Part model, mm, in its own coordinate system. A direction names the side the tool comes from. Round coordinates to 2 decimals unless told otherwise and drop trailing zeros. Loops run counter-clockwise (first coordinate to the right, second up) from the corner with the lowest first, then second, coordinate; pieces in that order, holes last. Notation, with made-up numbers: (57.25, 16.25) - (94.25, 16.25) arc R22 cw to (94.25, 50.25) - close; hole circle Ø1 at (60.5, 86.5). An arc over 180 degrees is marked (long way). Put each result on its own line as item: value.
from build123d import *

# Parameters (mm, degrees)
F1_DEPTH = 6.35


with BuildPart() as f1:
    # F0 (on Top) → F1 (new body)
    with BuildSketch(Plane.XY):
        with BuildLine():
            ThreePointArc((0, 11.049), (7.8128228253, 7.8128228253), (11.049, 0))
            ThreePointArc((11.049, 0), (7.8128228253, -7.8128228253), (0, -11.049))
            Line((0, -11.049), (0, -13.97))
            ThreePointArc((0, -13.97), (9.8782817332, -9.8782817332), (13.97, 0))
            ThreePointArc((13.97, 0), (9.8782817332, 9.8782817332), (0, 13.97))
            Line((0, 13.97), (0, 11.049))
        make_face()
        with BuildLine():
            ThreePointArc((0, -11.049), (-11.049, 0), (0, 11.049))
            Line((0, 11.049), (0, 13.97))
            ThreePointArc((0, 13.97), (-9.8782817332, 9.8782817332), (-13.97, 0))
            ThreePointArc((-13.97, 0), (-9.8782817332, -9.8782817332), (0, -13.97))
            Line((0, -13.97), (0, -11.049))
        make_face()
        with BuildLine():
            Line((0, 16.51), (0, 13.97))
            ThreePointArc((0, 13.97), (9.8782817332, 9.8782817332), (13.97, 0))
            Line((13.97, 0), (13.97, 30.48))
            ThreePointArc((13.97, 30.48), (9.8782817332, 20.6017182668), (0, 16.51))
        make_face()
        with BuildLine():
            ThreePointArc((-13.97, 0), (-9.8782817332, 9.8782817332), (0, 13.97))
            Line((0, 13.97), (0, 16.51))
            ThreePointArc((0, 16.51), (-9.8782817332, 20.6017182668), (-13.97, 30.48))
            Line((-13.97, 30.48), (-13.97, 0))
        make_face()
        with BuildLine():
            Line((0, -16.51), (0, -13.97))
            ThreePointArc((0, -13.97), (-9.8782817332, -9.8782817332), (-13.97, 0))
            Line((-13.97, 0), (-13.97, -30.48))
            ThreePointArc((-13.97, -30.48), (-9.8782817332, -20.6017182668), (0, -16.51))
        make_face()
        with BuildLine():
            ThreePointArc((13.97, 0), (9.8782817332, -9.8782817332), (0, -13.97))
            Line((0, -13.97), (0, -16.51))
            ThreePointArc((0, -16.51), (9.8782817332, -20.6017182668), (13.97, -30.48))
            Line((13.97, -30.48), (13.97, 0))
        make_face()
        with BuildLine():
            ThreePointArc((-13.97, 30.48), (-9.8782817332, 20.6017182668), (0, 16.51))
            ThreePointArc((0, 16.51), (9.8782817332, 20.6017182668), (13.97, 30.48))
            ThreePointArc((13.97, 30.48), (9.8782817459, 40.3582817204), (3.6e-08, 44.45))
            ThreePointArc((3.6e-08, 44.45), (-9.8782817204, 40.3582817459), (-13.97, 30.48))
        make_face()
        with BuildLine():
            ThreePointArc((11.049, 30.48), (7.8128228253, 22.6671771747), (0, 19.431))
            ThreePointArc((0, 19.431), (-7.8128228253, 38.2928228253), (11.049, 30.48))
        make_face(mode=Mode.SUBTRACT)
        with BuildLine():
            ThreePointArc((13.97, -30.48), (9.8782817332, -20.6017182668), (0, -16.51))
            ThreePointArc((0, -16.51), (-9.8782817332, -20.6017182668), (-13.97, -30.48))
            ThreePointArc((-13.97, -30.48), (-9.8782817062, -40.3582817602), (7.63e-08, -44.45))
            ThreePointArc((7.63e-08, -44.45), (9.8782817602, -40.3582817062), (13.97, -30.48))
        make_face()
        with BuildLine():
            ThreePointArc((11.049, -30.48), (-7.8128228253, -38.2928228253), (0, -19.431))
            ThreePointArc((0, -19.431), (7.8128228253, -22.6671771747), (11.049, -30.48))
        make_face(mode=Mode.SUBTRACT)
        with BuildLine():
            ThreePointArc((3.6e-08, 44.45), (9.8782817459, 40.3582817204), (13.97, 30.48))
            ThreePointArc((13.97, 30.48), (23.1619287876, 34.4165277907), (32.3538575753, 30.48))
            ThreePointArc((32.3538575753, 30.48), (17.6205349119, 40.808323286), (3.6e-08, 44.45))
        make_face()
        with BuildLine():
            ThreePointArc((32.3538575753, -30.48), (23.1619287876, -34.4165277907), (13.97, -30.48))
            ThreePointArc((13.97, -30.48), (9.8782817602, -40.3582817062), (7.63e-08, -44.45))
            ThreePointArc((7.63e-08, -44.45), (17.6205349304, -40.808323278), (32.3538575753, -30.48))
        make_face()
        with BuildLine():
            ThreePointArc((7.63e-08, -44.45), (-9.8782817062, -40.3582817602), (-13.97, -30.48))
            ThreePointArc((-13.97, -30.48), (-23.1619287876, -34.4165277907), (-32.3538575753, -30.48))
            ThreePointArc((-32.3538575753, -30.48), (-17.6205348604, -40.8083233083), (7.63e-08, -44.45))
        make_face()
        with BuildLine():
            ThreePointArc((-32.3538575753, 30.48), (-23.1619287876, 34.4165277907), (-13.97, 30.48))
            ThreePointArc((-13.97, 30.48), (-9.8782817204, 40.3582817459), (3.6e-08, 44.45))
            ThreePointArc((3.6e-08, 44.45), (-17.6205348789, 40.8083233003), (-32.3538575753, 30.48))
        make_face()
    extrude(amount=F1_DEPTH)


solid = f1.part
1. Pin check, flat tips, straight feed: P1, Ø2, axis at y = -14.5, z = 3, coming from the +X side; P2, Ø1.5, axis at x = 11.5, z = 4, coming from the +Y side; P3, Ø5, axis at x = 7.5, y = 34, coming from the +Z side; P4, Ø1, axis at x = 18, z = 5.5, coming from the -Y side. Stop position of each tip, or through.
A:
P1: stops at x = 13.97
P2: stops at y = 43.13
P3: passes through
P4: stops at y = -40.86
2. Probe line 1 along Y through (x, z) = (-2.5, 1); line 2 along X through (y, z) = (-32.5, 3); line 3 along Y through (x, z) = (-9.5, 4). List the from-to ranges inside material, lowest first. Write a range as [from, to].
A:
line 1: y = [-44.38, -41.24], [-19.72, -10.76], [10.76, 19.72], [41.24, 44.38]
line 2: x = [-30.32, -29.87], [-16.45, -10.86], [10.86, 16.45], [29.87, 30.32]
line 3: y = [-43.42, -36.12], [-24.84, -5.64], [5.64, 24.84], [36.12, 43.42]
3. Band-saw the part on A-A (y = 5). List the corners of the cut face in (x, z), plus the area to 3 significant figures.
A:
outline: (-13.97, 0) - (-9.85, 0) - (-9.85, 6.35) - (-13.97, 6.35) - close; (9.85, 0) - (13.97, 0) - (13.97, 6.35) - (9.85, 6.35) - close
area: 52.3 mm²
4. Two-plate mould, pull along Y, no slides. Class faces 1 (the flat face through (13.97, 0, 3)), 2 (the cylindrical face through (23.018, 34.416, 3.131)), 3 (the flat face through (-10, -6, 0)): pulls with the +Y half, pulls with the -Y half, needs draft (parallel to the pull), parting line crosses it, or undercut.
A:
face 1: undercut
face 2: undercut
face 3: needs draft
5. Tool access for faces 4 (the flat face through (-13.97, 0, 3)), 5 (the flat face through (-10, -6, 6.35)), 6 (the cylindrical face through (23.306, -34.416, 3.131)): list every direction of +Z, -Z, +X, -X, +Y, -Y with a clear straight run to the whole face (end or side of a thin tool).
A:
face 4: +Z, -Z, -X
face 5: +Z, +X, -X, +Y, -Y
face 6: +Z, -Z
6. Band-saw the part on C-C (y = -32). List the corners of the cut face in (x, z), plus the area to 3 significant figures.
A:
outline: (-30.85, 0) - (-30.61, 0) - (-30.61, 6.35) - (-30.85, 6.35) - close; (-15.71, 0) - (-10.94, 0) - (-10.94, 6.35) - (-15.71, 6.35) - close; (10.94, 0) - (15.71, 0) - (15.71, 6.35) - (10.94, 6.35) - close; (30.61, 0) - (30.85, 0) - (30.85, 6.35) - (30.61, 6.35) - close
area: 63.5 mm²
7. Band-saw the part on B-B (z = 2.5). List the corners of the cut face in (x, y), plus the area to 3 significant figures.
A:
outline: (-32.35, -30.48) arc R44.45 ccw to (32.35, -30.48) arc R12.7 cw to (13.97, -30.48) - (13.97, 30.48) arc R12.7 cw to (32.35, 30.48) arc R44.45 ccw to (-32.35, 30.48) arc R12.7 cw to (-13.97, 30.48) - (-13.97, -30.48) arc R12.7 cw to start; hole circle Ø22.1 at (0, -30.48); hole circle Ø22.1 at (0, 0); hole circle Ø22.1 at (0, 30.48)
area: 1,600 mm²
8. Band-saw the part on D-D (x = -4). List the corners of the cut face in (y, z), plus the area to 3 significant figures.
A:
outline: (-44.27, 0) - (-40.78, 0) - (-40.78, 6.35) - (-44.27, 6.35) - close; (-20.18, 0) - (-10.3, 0) - (-10.3, 6.35) - (-20.18, 6.35) - close; (10.3, 0) - (20.18, 0) - (20.18, 6.35) - (10.3, 6.35) - close; (40.78, 0) - (44.27, 0) - (44.27, 6.35) - (40.78, 6.35) - close
area: 170 mm²
